Autodesk Inventor part; units mm, degrees
ref_plane "YZ Plane" through (0, 0, 0) normal (1, 0, 0) x (0, 1, 0)
ref_plane "XZ Plane" through (0, 0, 0) normal (0, 1, 0) x (-1, 0, 0)
ref_plane "XY Plane" through (0, 0, 0) normal (0, 0, 1) x (1, 0, 0)
sketch "Skizze1" plane through (0, 0, 0) normal (0, 1, 0) x (-1, 0, 0)
  line L0 (0, 0) -> (42.3, 0)
  line L1 (42.3, 0) -> (42.3, -42.3)
  line L2 (42.3, -42.3) -> (0, -42.3)
  line L3 (0, -42.3) -> (0, 0)
  dimension "d0" = 42.3
  dimension "d1" = 42.3
extrude "Extrusion1" add sketch "Skizze1" along normal blind 47
sketch "Skizze2" plane through (0, 47, 0) normal (0, 1, 0) x (1, 0, 0)
  line L0 (-42.3, 42.3) -> (-42.3, 0)
  line L1 (-42.3, 21.15) -> (0, 21.15)
  line L2 (0, 0) -> (0, 42.3)
  line L3 (-42.3, 0) -> (0, 0)
  line L4 (-21.15, 0) -> (-21.15, 42.3)
  line L5 (0, 42.3) -> (-42.3, 42.3)
  circle A0 centre (-21.15, 21.15) radius 5
  dimension "d4" = 10
extrude "Extrusion2" cut sketch "Skizze2" against normal blind 47 contours A0 L4 L1 | L1 L4 A0 | A0 L1 L4 | L1 A0 L4
properties part number "Motor"
Here's how the part is built. I have some questions about the finished solid (model axes, mm). Coordinates: 2 decimals unless noted, no trailing zeros. Loops run counter-clockwise (first coordinate to the right, second up) from the corner with the lowest first, then second, coordinate; pieces in that order, holes last.
1. If we mould it in two halves opening along X, with no side actions, what happens to faces 1 (the flat face through (-42.3, 23, -21)), 2 (the flat face through (0, 23, -21)), 3 (the cylindrical face through (-24.835, 23.829, -24.529)), 4 (the flat face through (-21, 23, -42.3))? For each: pulls with the +X half, pulls with the -X half, needs draft (parallel to the pull), parting line crosses it, or undercut.
2. Imagine slicing it at C-C, the plane z = -21.15. Please give me the cut outline in (x, y), and give its area (3 significant figures).
3. I need wall thicknesses on L1, parallel to Z at x = -21, y = 25; L2, parallel to X at y = 14.5, z = -23. Which ranges of each line are inside material? Lowest first, please.
4. Imagine slicing it at A-A, the plane x = -21.15. Please give me the cut outline in (y, z).
5. Imagine slicing it at B-B, the plane y = 5. Please give me the cut outline in (x, z).
Taken from the geometry:
1. face 1: pulls with the -X half
1. face 2: pulls with the +X half
1. face 3: undercut
1. face 4: needs draft
2. outline: (-42.3, 0) - (-26.15, 0) - (-26.15, 47) - (-42.3, 47) - close; (-16.15, 0) - (0, 0) - (0, 47) - (-16.15, 47) - close
2. area: 1,520 mm2
3. L1: z = -42.3 to -26.15, -16.15 to 0
3. L2: x = -42.3 to -25.8, -16.5 to 0
4. outline: (0, -42.3) - (47, -42.3) - (47, -26.15) - (0, -26.15) - close; (0, -16.15) - (47, -16.15) - (47, 0) - (0, 0) - close
5. outline: (-42.3, -42.3) - (0, -42.3) - (0, 0) - (-42.3, 0) - close; hole circle Ø10 at (-21.15, -21.15)
